The drawing under review shows one solid part. Ordinate dimensions are in mm from its lowest x, y, z. A direction names the side the tool comes from. Give positions to 0.01 mm unless a question says otherwise; leave off trailing zeros. Write each loop counter-clockwise with the first axis right and the second up, starting at its lowest first coordinate (ties: lowest second). Pieces come first, ordered by that corner, then holes. Notation, with made-up numbers: (31, 50) -> (61, 50) arc R17 ccw to (61, 81) -> close; hole circle Ø4 at (49.25, 75.25). An arc over 180 degrees is marked (long way). Answer as a JSON object with one key per item and string values.
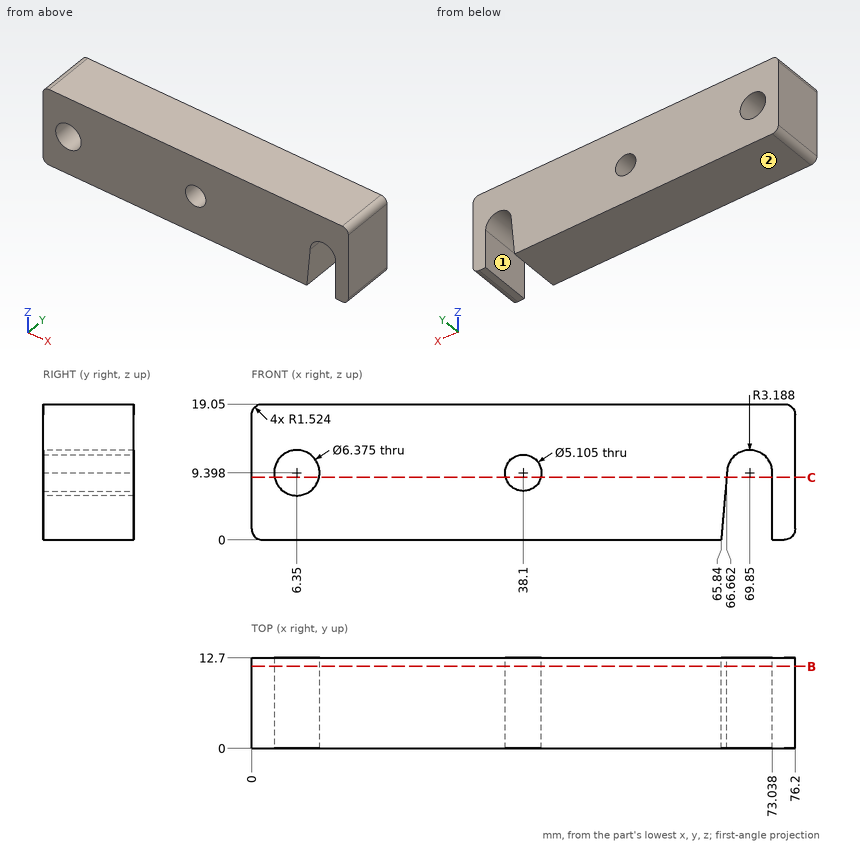
(1) For line 1 along X through (y, z) = (9.5, 6.5) (1 decimal); line 2 along X through (y, z) = (7.25, 6.75) (1 decimal); line 3 along X through (y, z) = (8.5, 10.5), list the stretches that pass through material, from the lowest coordinate up.
Here are the results:
{"line 1": "x = 0 to 5, 7.7 to 66.4, 73 to 76.2", "line 2": "x = 0 to 4.6, 8.1 to 66.4, 73 to 76.2", "line 3": "x = 0 to 3.36, 9.34 to 35.8, 40.4 to 66.86, 72.84 to 76.2"}
(2) Clearance check with flat-ended pins moving along their axes: pin 1 (7.5 mm diameter, centred on x = 6.35, z = 9.398, fed in from -Y); pin 2 (4.5 mm diameter, centred on x = 38.1, z = 9.398, fed in from -Y). State where each tip first meets the part, or that it passes through.
Here are the results:
{"pin 1": "stops at y = 0", "pin 2": "passes through"}
(3) We need section C-C, the plane z = 8.75. State the section outline as (x, y) points (1 decimal), then the cut area to 3 significant figures.
Here are the results:
{"outline": "(0, 0) -> (3.2, 0) -> (3.2, 12.7) -> (0, 12.7) -> close; (9.5, 0) -> (35.6, 0) -> (35.6, 12.7) -> (9.5, 12.7) -> close; (40.6, 0) -> (66.6, 0) -> (66.6, 12.7) -> (40.6, 12.7) -> close; (73, 0) -> (76.2, 0) -> (76.2, 12.7) -> (73, 12.7) -> close", "area": "744 mm²"}
(4) We need section B-B, the plane y = 11.5. Give the number of separate pieces and of enclosed holes in the cut face, then the cut area to 3 significant figures.
Here are the results:
{"separate pieces": "1", "enclosed holes": "2", "area": "1,320 mm²"}
(5) For the marked faces 1 and 2, list the 3-axis set-ups (+Z, -Z, +X, -X, +Y, -Y) from which the entire face can be reached by the end or side of a thin tool; tool diameter is ignored.
Here are the results:
{"face 1": "-Z, +Y, -Y", "face 2": "-Z, +X, -X, +Y, -Y"}
